Read the model definition and answer for the solid it produces. Units are mm, in the model's axes. Face numbers are marked on the shaded views. A direction names the side the tool comes from. Coordinates: 2 decimals unless noted, no trailing zeros. Write each loop counter-clockwise with the first axis right and the second up, starting at its lowest first coordinate (ties: lowest second). Pieces come first, ordered by that corner, then holes. Notation, with made-up numbers: (85.5, 9) -> (131.5, 9) arc R25 ccw to (131.5, 44) -> close; hole circle Ø3 at (65, 51). An arc over 180 degrees is marked (long way). One line per item, written item: value. Start each with the question number.
from build123d import *

# Parameters (mm, degrees)
CYLINDER024_R                      = 2
CYLINDER024_DEPTH                  = 22.8
CYLINDER023_R                      = 3.5
CYLINDER023_DEPTH                  = 2.8
FUSION001018017022_PLACEMENT_ANGLE = 180
POCKET002018004005005_DEPTH        = 2.5


with BuildPart() as cylinder024:
    # Cylinder024 → Cylinder024 (new body)
    with BuildSketch(Plane.XY):
        Circle(CYLINDER024_R)
    extrude(amount=CYLINDER024_DEPTH)


with BuildPart() as obj1:
    # Cylinder023 → Cylinder023 (new body)
    with BuildSketch(Plane.XY):
        Circle(CYLINDER023_R)
    extrude(amount=CYLINDER023_DEPTH)

    # Fusion001018017022: union Cylinder024
    add(cylinder024.part)


with BuildPart() as obj1_1:
    # Fusion001018017022 placement: moved
    add(obj1.part.rotate(Axis((0, 0, 0), (0, 1, 0)), FUSION001018017022_PLACEMENT_ANGLE))

    # Sketch023 → Pocket002018004005005 (cut)
    with BuildSketch(Plane(origin=(0, 0, 0), x_dir=(-1, 0, 0), z_dir=(0, 0, 1))):
        Polygon((1.5, -0.866025), (1.5, 0.866025), (0, 1.732051), (-1.5, 0.866025), (-1.5, -0.866025), (0, -1.732051), align=None)
    extrude(amount=-POCKET002018004005005_DEPTH, mode=Mode.SUBTRACT)


solid = obj1_1.part
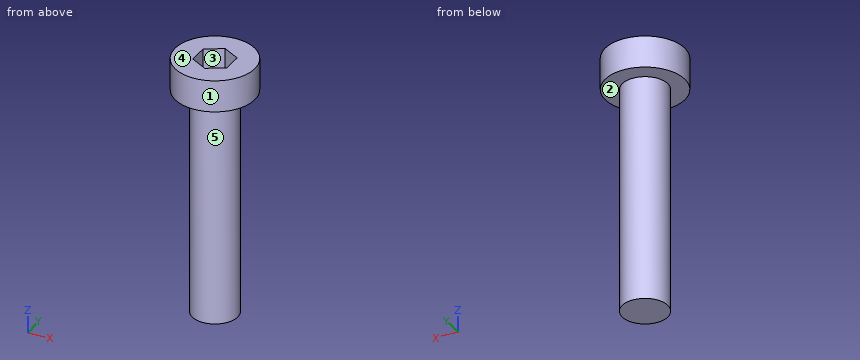
1. A cutting plane is placed at C-C on x = -1. Give the vertices of the cut face in (y, z), then the cut area to 3 significant figures.
2. A cutting plane is placed at A-A on y = 0. Give the vertices of the cut face in (x, z), then the cut area to 3 significant figures.
3. Given pin 1 (3 mm diameter, centred on x = -2, z = -19, fed in from +Y); pin 2 (4 mm diameter, centred on x = 2.5, z = -8, fed in from -Y), each flat-ended and moving along its own axis, determine where each tip first touches the part or whether it passes through.
4. Find the intervals of material crossed by probe 1 along X at (y, z) = (-1, -20.75); probe 2 along Z at (x, y) = (3, 0.5), in increasing order. Write a range as from..to.
5. For a pull along X with two mould halves and no side action, classify the marked faces 3, 4 and 5 as +X half, -X half, draft (parallel to the pull), parting line (faces both ways), or undercut.
6. A cutting plane is placed at B-B on z = -20.25. Give the vertices of the cut face in (x, y), then the cut area to 3 significant figures.
7. A tool of negligible diameter and unlimited length cuts with its end or side. For the marked faces 1 and 2, from which of +Z, -Z, +X, -X, +Y, -Y can it reach the whole face along a straight path? Write none if from no direction.
Derived:
1. outline: (-3.35, -2.8) -> (-1.73, -2.8) -> (-1.73, -22.8) -> (1.73, -22.8) -> (1.73, -2.8) -> (3.35, -2.8) -> (3.35, 0) -> (1.15, 0) -> (1.15, -2.5) -> (-1.15, -2.5) -> (-1.15, 0) -> (-3.35, 0) -> close
1. area: 82.3 mm2
2. outline: (-3.5, -2.8) -> (-2, -2.8) -> (-2, -22.8) -> (2, -22.8) -> (2, -2.8) -> (3.5, -2.8) -> (3.5, 0) -> (1.5, 0) -> (1.5, -2.5) -> (-1.5, -2.5) -> (-1.5, 0) -> (-3.5, 0) -> close
2. area: 92.1 mm2
3. pin 1: stops at y = 1.94
3. pin 2: stops at y = -1.94
4. probe 1: x = -1.73..1.73
4. probe 2: z = -2.8..0
5. face 3: undercut
5. face 4: draft
5. face 5: parting line
6. outline: circle Ø4 at (0, 0)
6. area: 12.6 mm2
7. face 1: +Z, -Z
7. face 2: -Z
